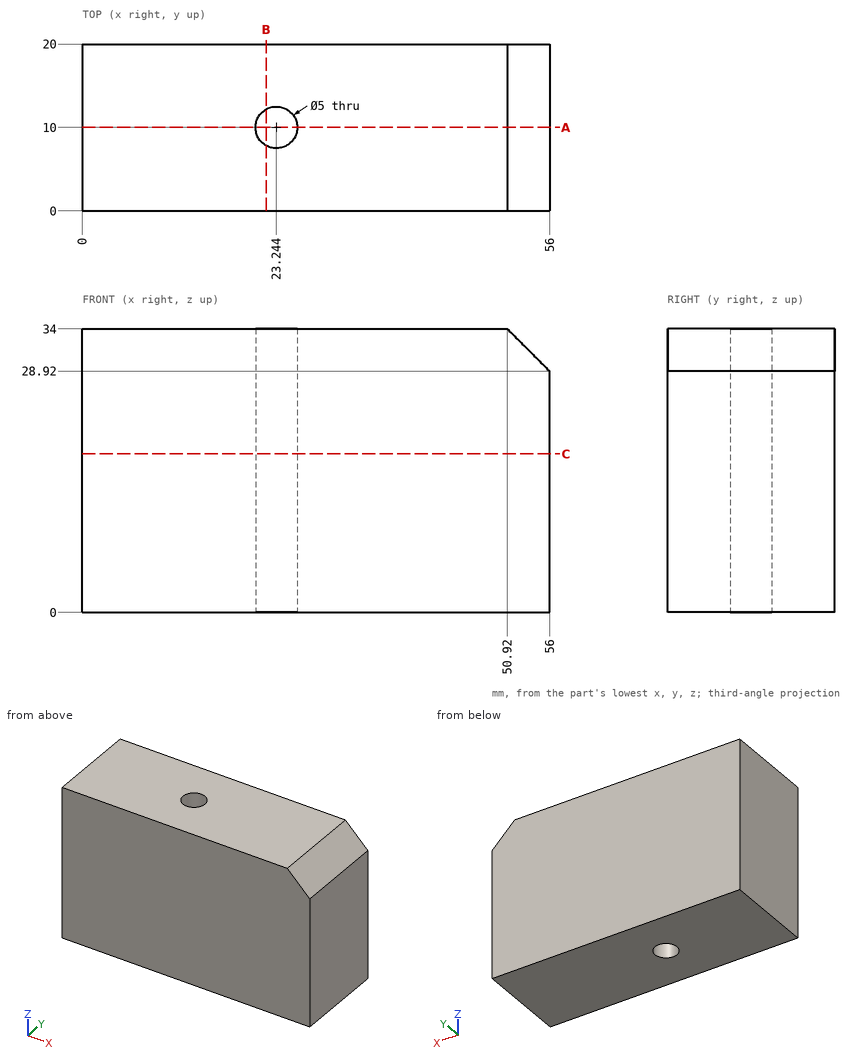
Can you work these out from the drawing? Everything is in mm from the part's minimum corner. Coordinates: 2 decimals unless noted, no trailing zeros. Loops run counter-clockwise (first coordinate to the right, second up) from the corner with the lowest first, then second, coordinate; pieces in that order, holes last.
1. Imagine slicing it at C-C, the plane z = 19. Please give me the cut outline in (x, y), and give its area (3 significant figures).
2. I need wall thicknesses on L1, parallel to Y at x = 22.5, z = 18; L2, parallel to X at y = 8, z = 6 (1 decimal); L3, parallel to X at y = 14.25, z = 32.5. Which ranges of each line are inside material? Lowest first, please.
3. Imagine slicing it at B-B, the plane x = 22. Please give me the cut outline in (y, z).
4. Imagine slicing it at A-A, the plane y = 10. Please give me the cut outline in (x, z), and give its area (3 significant figures).
Taken from the geometry:
1. outline: (0, 0) - (56, 0) - (56, 20) - (0, 20) - close; hole circle Ø5 at (23.24, 10)
1. area: 1,100 mm2
2. L1: y = 0 to 7.61, 12.39 to 20
2. L2: x = 0 to 21.7, 24.7 to 56
2. L3: x = 0 to 52.42
3. outline: (0, 0) - (7.83, 0) - (7.83, 34) - (0, 34) - close; (12.17, 0) - (20, 0) - (20, 34) - (12.17, 34) - close
4. outline: (0, 0) - (20.74, 0) - (20.74, 34) - (0, 34) - close; (25.74, 0) - (56, 0) - (56, 28.92) - (50.92, 34) - (25.74, 34) - close
4. area: 1,720 mm2
